Verification items for the finished model (mm, model axes). A direction names the side the tool comes from. Round coordinates to 2 decimals unless told otherwise and drop trailing zeros. Order: outer loops, then holes, each group sorted by start corner. A loop starts at its lowest first (then second) coordinate and runs counter-clockwise, first axis right, second up. Notation, with made-up numbers: M 58,-13.5 L 109,-13.5 A20 cw 109,-4.5 Z; hole C 42,65 d9. An arc over 180 degrees is marked long. Use one line per item in the form item = value. Start each with the question number.
Item 1: Thickness scan on probe 1 along Y at (x, z) = (0.95, -17.5); probe 2 along Y at (x, z) = (11, -16.25); probe 3 along X at (y, z) = (18, -10.25). Record the ranges inside material, lowest first. Write a range as [from, to].
Item 2: Cross-section at B-B on z = -2.5. Enter the section's corners in (x, y).
Item 3: Cross-section at D-D on y = 12.5. Enter the section's corners in (x, z).
Item 4: Go/stop test with flat-tipped pins: pin 1 Ø2 at (x, y) = (10, 6) entering from +Z; pin 2 Ø8 at (x, z) = (8, -10) entering from -Y; pin 3 Ø3 at (x, y) = (10.5, 6.5) entering from -Z. Record where each tip stops, or that it passes through.
Item 5: Tool access check on faces 1 (the flat face through (8, 4.572, -10)), 2 (the flat face through (8, 6, -16.571)), 3 (the flat face through (8, 7.112, -10)), 4 (the flat face through (8, 6, -3.414)). Record the directions out of +Z, -Z, +X, -X, +Y, -Y that give a thin tool (end or side, any length) a straight path to the whole face; none if there is none.
Item 6: Cross-section at A-A on y = 2.5. Enter the section's corners in (x, z), then the cut area to 3 significant figures.
Item 7: Cross-section at C-C on z = -7. Enter the section's corners in (x, y), then the cut area to 3 significant figures.
from build123d import *

# Parameters (mm, degrees)
SKETCH1_W          = 20
SKETCH1_H          = 20
EXTRUDE1_DEPTH     = 1.6002
SKETCH2_R          = 1.4224
CUT_EXTRUDE1_DEPTH = 2.6002
SKETCH3_W          = 13.1572
SKETCH3_H          = 2.54
EXTRUDE2_DEPTH     = 12.7


with BuildPart() as part:
    # Sketch1 → Extrude1 (new body)
    with BuildSketch(Plane(origin=(0, 0, 0), x_dir=(0, 0, -1), z_dir=(1, 0, 0))):
        with Locations((10, 10)):
            Rectangle(SKETCH1_W, SKETCH1_H)
    extrude(amount=EXTRUDE1_DEPTH)

    # Sketch2 → Cut-Extrude1 (cut, through all)
    with BuildSketch(Plane(origin=(1.6002, 0, 0), x_dir=(0, 0, -1), z_dir=(1, 0, 0))):
        with Locations((2.5, 17.5)):
            Circle(SKETCH2_R)
        with Locations((17.5, 17.5)):
            Circle(SKETCH2_R)
        with Locations((17.5, 2.5)):
            Circle(SKETCH2_R)
        with Locations((2.5, 2.5)):
            Circle(SKETCH2_R)
    extrude(amount=-CUT_EXTRUDE1_DEPTH, mode=Mode.SUBTRACT)

    # Sketch3 → Extrude2 (add)
    with BuildSketch(Plane(origin=(1.6002, 0, 0), x_dir=(0, 0, -1), z_dir=(1, 0, 0))):
        with Locations((9.9924, 5.842)):
            Rectangle(SKETCH3_W, SKETCH3_H)
    extrude(amount=EXTRUDE2_DEPTH)


solid = part.part
Output values:
q1.probe_1 = [0, 1.08], [3.92, 16.08], [18.92, 20]
q1.probe_2 = [4.57, 7.11]
q1.probe_3 = [0, 1.6]
q2.outline = M 0,0 L 1.6,0 L 1.6,1.08 L 0,1.08 Z; M 0,3.92 L 1.6,3.92 L 1.6,16.08 L 0,16.08 Z; M 0,18.92 L 1.6,18.92 L 1.6,20 L 0,20 Z
q3.outline = M 0,-20 L 1.6,-20 L 1.6,0 L 0,0 Z
q4.pin_1 = -3.41
q4.pin_2 = 4.57
q4.pin_3 = -16.57
q5.face_1 = +Z, -Z, +X, -Y
q5.face_2 = -Z, +X, +Y, -Y
q5.face_3 = +Z, -Z, +X, +Y
q5.face_4 = +Z, +X, +Y, -Y
q6.outline = M 0,-20 L 1.6,-20 L 1.6,-18.92 L 0,-18.92 Z; M 0,-16.08 L 1.6,-16.08 L 1.6,-3.92 L 0,-3.92 Z; M 0,-1.08 L 1.6,-1.08 L 1.6,0 L 0,0 Z
q6.area = 22.9 mm2
q7.outline = M 0,0 L 1.6,0 L 1.6,4.57 L 14.3,4.57 L 14.3,7.11 L 1.6,7.11 L 1.6,20 L 0,20 Z
q7.area = 64.3 mm2
